Design review of the part built by this model. Coordinates are the model's own, in mm. A direction names the side the tool comes from. Round coordinates to 2 decimals unless told otherwise and drop trailing zeros. Write each loop counter-clockwise with the first axis right and the second up, starting at its lowest first coordinate (ties: lowest second). Pieces come first, ordered by that corner, then holes. Notation, with made-up numbers: (8, 63.5) - (29, 63.5) arc R5 ccw to (29, 71.5) - close; hole circle Ø5 at (-13.75, 20). An arc over 180 degrees is marked (long way). Use one line per item in the form item = value.
```python
from build123d import *

# Parameters (mm, degrees)
F0_R        = 7.25
F1_DEPTH    = 30
F3_DEPTH    = 4.7
F4_T1_DEPTH = 22.95
F4_T3_DEPTH = 23.089756942
F5_SIZE2    = 4
F5_SIZE     = 5
F6_SIZE2    = 3
F6_SIZE     = 4.5
F7_SIZE     = 5
F8_SIZE     = 3


# Not quite as in the source:
# - a fillet or chamfer that OpenCascade refuses, or shapes differently, is made with other operations: its cross-section is extruded or revolved along the edge and cut away or added


with BuildPart() as f1:
    # F0 (on Front) → F1 (new body)
    with BuildSketch(Plane.XZ):
        Circle(F0_R)
    extrude(amount=F1_DEPTH)

    # F2 (on face) → F3 (join)
    with BuildSketch(Plane(origin=(0, 0, 0), x_dir=(-1, 0, 0), z_dir=(0, 1, 0))):
        Polygon((20.0881361961, 7.1568624116), (7.2347377427, 7.3653035797), (-7.2347377427, 7.3653035797), (-7.2347377427, -7.3653035797), (7.2347377427, -7.2549186188), (20.0881361961, -7.1568624116), align=None)
        Polygon((7.2347377427, 15.7034024596), (7.2347377427, 7.3653035797), (20.0881361961, 7.1568624116), (20.0881361961, 15.7034024596), align=None)
        Polygon((20.0881361961, -15.8427814022), (20.0881361961, -7.1568624116), (7.2347377427, -7.2549186188), (7.2347377427, -15.8427814022), align=None)
    extrude(amount=F3_DEPTH)

    # F4: fillet of radius 7.3 on 2 edges, made by hand

    # F4_s2 → F4_t1 (cut)
    with BuildSketch(Plane.XZ.offset(-22.95)):
        with BuildLine():
            ThreePointArc((7.2347377427, 0.0653035797), (5.0966172454, 5.2271830824), (-0.0652622573, 7.3653035797))
            Line((-0.0652622573, 7.3653035797), (7.2347377427, 7.3653035797))
            Line((7.2347377427, 7.3653035797), (7.2347377427, 0.0653035797))
        make_face()
    extrude(amount=F4_T1_DEPTH, mode=Mode.SUBTRACT)

    # F4_s4 → F4_t3 (cut)
    with BuildSketch(Plane.XZ.offset(-23.089756942)):
        with BuildLine():
            ThreePointArc((7.2347377427, -0.0094008029), (5.0768906111, -5.190931839), (-0.120950991, -7.3091883865))
            Line((-0.120950991, -7.3091883865), (7.2347377427, -7.3653035797))
            Line((7.2347377427, -7.3653035797), (7.2347377427, -0.0094008029))
        make_face()
    extrude(amount=F4_T3_DEPTH, mode=Mode.SUBTRACT)

    # F5
    f5_edges = [f1.edges().sort_by_distance(p)[0] for p in [
        (5.096617, 4.7, 5.227183),
        (5.076891, 4.7, -5.190932),
    ]]
    chamfer(f5_edges, length=F5_SIZE, length2=F5_SIZE2)

    # F6
    f6_edges = [f1.edges().sort_by_distance(p)[0] for p in [
        (-20.088136, 4.7, -0.069689),
    ]]
    f6_side = f1.faces().sort_by_distance((-20.088136, 2.35, -0.069689))[0]
    chamfer(f6_edges, length=F6_SIZE, length2=F6_SIZE2, reference=f6_side)

    # F7
    f7_edges = [f1.edges().sort_by_distance(p)[0] for p in [
        (-7.25, -30, 0),
    ]]
    chamfer(f7_edges, length=F7_SIZE)

    # F8
    f8_edges = [f1.edges().sort_by_distance(p)[0] for p in [
        (-7.234738, 4.7, 11.534353),
        (-7.234738, 4.7, -11.54885),
    ]]
    chamfer(f8_edges, length=F8_SIZE)


solid = f1.part
```
Q1. For P1, Ø1.5, axis at x = -6.5, y = -22, coming from the +Z side; P2, Ø0.6, axis at x = 7, z = -1.5, coming from the +Y side; P3, Ø4, axis at x = -3, y = -4, coming from the +Z side; P4, Ø1.5, axis at x = -9, y = -7.5, coming from the +Z side, all flat-tipped, find the tip position at first contact; note any pin that passes through.
Calculated:
P1 = 4.42
P2 = 1
P3 = 7.18
P4 = through
Q2. To check wall thickness, follow line 1 along Z through (x, y) = (-0.25, -14.5); line 2 along Y through (x, z) = (-9.5, -4.5); line 3 along Z through (x, y) = (0, 3.5). State the ranges of each line that lie inside material, in increasing order. Write a range as from..to.
Calculated:
line_1 = -7.25..7.25
line_2 = 0..3.97
line_3 = -3.81..3.86
Q3. We need section C-C on x = -13.75. Write out the cut boundary in (y, z).
Calculated:
outline = (0, -15.84) - (4.7, -15.84) - (4.7, 15.7) - (0, 15.7) - close
Q4. We need section B-B on y = -23.5. Write out the cut boundary in (x, z), then the cut area to 3 significant figures.
Calculated:
outline = circle Ø14.5 at (0, 0)
area = 165 mm2
Q5. Machinability: for faces 1 (the flat face through (-8.756, 3.221, 10.423)), 2 (the flat face through (-14, 2, -15.843)), 3 (the cylindrical face through (3.35, -12.32, -6.43)), which of the approach directions +Z, -Z, +X, -X, +Y, -Y give a long, thin tool a straight path to every point of the face, cutting with its end or side? Answer none if there is none.
Calculated:
face_1 = +Z, +X, +Y
face_2 = -Z, +X, -X, +Y, -Y
face_3 = -Y
Q6. We need section A-A on z = -12. Write out the cut boundary in (x, y).
Calculated:
outline = (-20.09, 0) - (-7.23, 0) - (-7.23, 1.7) - (-10.23, 4.7) - (-17.09, 4.7) - (-20.09, 0.2) - close
